For this review, take the finished solid that the model builds, in its own axes (mm). Face numbers are marked on the shaded views. A direction names the side the tool comes from. Give positions to 0.01 mm unless a question says otherwise; leave off trailing zeros. Write each loop counter-clockwise with the first axis right and the second up, starting at its lowest first coordinate (ties: lowest second). Pieces come first, ordered by that corner, then holes.
1) Draft analysis for pull direction X (two halves, no side actions). For the marked faces 4, 5, 6 and 7, state which applies: pulls with the +X half, pulls with the -X half, needs draft (parallel to the pull), parting line crosses it, or undercut.
2) We need section A-A on x = -221. Give the boundary of the cut face in (y, z), and give its area (3 significant figures).
3) For P1, Ø3, axis at x = -159, y = 22.5, coming from the +Z side; P2, Ø3.5, axis at y = 38.43, z = -27.92, coming from the +X side; P3, Ø12, axis at x = -80, z = -32, coming from the +Y side; P4, Ø17, axis at y = 8, z = 8, coming from the -X side, all flat-tipped, find the tip position at first contact; note any pin that passes through.
4) Wall thickness on line 1 along Y through (x, z) = (-251, 0); line 2 along Y through (x, z) = (-6, 0); line 3 along X through (y, z) = (-34, -6): over which ranges is each line inside the solid? List them lowest first.
5) Machinability: for the marked faces 1, 2 and 3, which of the approach directions +Z, -Z, +X, -X, +Y, -Y give a long, thin tool a straight path to every point of the face, cutting with its end or side? Answer none if there is none.
6) We need section B-B on x = -193. Give the boundary of the cut face in (y, z), and give its area (3 significant figures).
from build123d import *

# Parameters (mm, degrees)
SKETCH2_R          = 2
CUT_EXTRUDE1_DEPTH = 10
SKETCH3_R          = 2
CUT_EXTRUDE2_DEPTH = 10


with BuildPart() as part:
    # Sketch1 → Revolve1 (revolve)
    with BuildSketch(Plane.XY, mode=Mode.PRIVATE) as revolve1_sk:
        with BuildLine():
            Line((-13.547676843, 80), (-3.547676843, 80))
            Line((-3.547676843, 80), (-3.547676843, 120))
            Line((-3.547676843, 120), (-6.547676843, 120))
            Line((-6.547676843, 120), (-6.547676843, 117.5))
            Line((-6.547676843, 117.5), (-26.547676843, 117.5))
            Line((-26.547676843, 117.5), (-26.547676843, 119.563264874))
            ThreePointArc((-26.547676843, 119.563264874), (-46.73701782, 116.53049781), (-66.547676843, 111.59643719))
            Line((-66.547676843, 111.59643719), (-66.547676843, 104.5))
            Line((-66.547676843, 104.5), (-86.547676843, 104.5))
            ThreePointArc((-86.547676843, 104.5), (-107.122168132, 94.730106924), (-126.547676843, 82.838508469))
            Line((-126.547676843, 82.838508469), (-126.547676843, 75))
            Line((-126.547676843, 75), (-146.547676843, 75))
            Line((-146.547676843, 75), (-146.547676843, 67.275434145))
            ThreePointArc((-146.547676843, 67.275434145), (-165.253477075, 48.712256642), (-181.547676843, 28))
            Line((-181.547676843, 28), (-184.047676843, 28))
            Line((-184.047676843, 28), (-184.047676843, 26))
            Line((-184.047676843, 26), (-204.047676843, 26))
            Line((-204.047676843, 26), (-204.047676843, 28))
            Line((-204.047676843, 28), (-206.547676843, 28))
            Line((-206.547676843, 28), (-231.547676843, 55))
            Line((-231.547676843, 55), (-234.047676843, 55))
            Line((-234.047676843, 55), (-234.047676843, 53))
            Line((-234.047676843, 53), (-254.047676843, 53))
            Line((-254.047676843, 53), (-254.047676843, 55))
            Line((-254.047676843, 55), (-256.547676843, 55))
            Line((-256.547676843, 55), (-256.547676843, 30))
            Line((-256.547676843, 30), (-246.547676843, 30))
            Line((-246.547676843, 30), (-246.547676843, 45.820294157))
            Line((-246.547676843, 45.820294157), (-236.547676843, 45.820294157))
            Line((-236.547676843, 45.820294157), (-212.639997068, 20))
            Line((-212.639997068, 20), (-175.547676843, 20))
            ThreePointArc((-175.547676843, 20), (-105.298190774, 84.350925075), (-13.547676843, 110))
            Line((-13.547676843, 110), (-13.547676843, 80))
        make_face()
    revolve(revolve1_sk.sketch.rotate(Axis((-129.761904762, 0, 0), (1, 0, 0)), 90), axis=Axis((-129.761904762, 0, 0), (1, 0, 0)))

    # Sketch2 → Cut-Extrude1 (cut)
    with BuildSketch(Plane(origin=(-3.547676843, 0, 0), x_dir=(0, 0, -1), z_dir=(1, 0, 0))):
        with Locations((0, 92)):
            Circle(SKETCH2_R)
        with Locations((54.076243211, 74.429563482)):
            Circle(SKETCH2_R)
        with Locations((87.497199499, 28.429563482)):
            Circle(SKETCH2_R)
        with Locations((87.497199499, -28.429563482)):
            Circle(SKETCH2_R)
        with Locations((54.076243211, -74.429563482)):
            Circle(SKETCH2_R)
        with Locations((0, -92)):
            Circle(SKETCH2_R)
        with Locations((-54.076243211, -74.429563482)):
            Circle(SKETCH2_R)
        with Locations((-87.497199499, -28.429563482)):
            Circle(SKETCH2_R)
        with Locations((-87.497199499, 28.429563482)):
            Circle(SKETCH2_R)
        with Locations((-54.076243211, 74.429563482)):
            Circle(SKETCH2_R)
    extrude(amount=-CUT_EXTRUDE1_DEPTH, mode=Mode.SUBTRACT)

    # Sketch3 → Cut-Extrude2 (cut)
    with BuildSketch(Plane.ZY.offset(256.547676843)):
        with Locations((0, 47.5)):
            Circle(SKETCH3_R)
        with Locations((27.919799484, 38.428307233)):
            Circle(SKETCH3_R)
        with Locations((45.175184524, 14.678307233)):
            Circle(SKETCH3_R)
        with Locations((45.175184524, -14.678307233)):
            Circle(SKETCH3_R)
        with Locations((27.919799484, -38.428307233)):
            Circle(SKETCH3_R)
        with Locations((0, -47.5)):
            Circle(SKETCH3_R)
        with Locations((-27.919799484, -38.428307233)):
            Circle(SKETCH3_R)
        with Locations((-45.175184524, -14.678307233)):
            Circle(SKETCH3_R)
        with Locations((-45.175184524, 14.678307233)):
            Circle(SKETCH3_R)
        with Locations((-27.919799484, 38.428307233)):
            Circle(SKETCH3_R)
    extrude(amount=-CUT_EXTRUDE2_DEPTH, mode=Mode.SUBTRACT)


solid = part.part
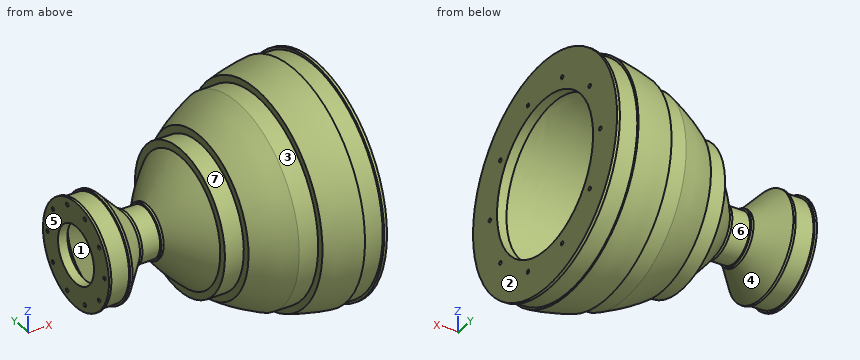
Results list:
1. face 4: undercut
1. face 5: pulls with the -X half
1. face 6: undercut
1. face 7: needs draft
2. outline: circle Ø87.22 at (0, 0); hole circle Ø58.06 at (0, 0)
2. area: 3,330 mm2
3. P1: stops at z = 52.45
3. P2: stops at x = -151.55
3. P3: stops at y = 101.21
3. P4: passes through
4. line 1: y = -53 to -49.5, -45.5 to -30, 30 to 45.5, 49.5 to 53
4. line 2: y = -120 to -94, -90 to -80, 80 to 90, 94 to 120
4. line 3: x = -256.55 to -246.55, -226.09 to -212.59, -176.85 to -164.76
5. face 1: none
5. face 2: +Z, -Z, +X, +Y, -Y
5. face 3: -X
6. outline: circle Ø52 at (0, 0); hole circle Ø40 at (0, 0)
6. area: 867 mm2
